Can you work these out from the model? Positions are in its coordinate system, mm. Face numbers are marked on the shaded views. Round coordinates to 2 decimals unless told otherwise and drop trailing zeros. Loops run counter-clockwise (first coordinate to the right, second up) from the corner with the lowest first, then second, coordinate; pieces in that order, holes last.
(1) I want a section at A-A on x = 152. Write out the boundary of the cut face in (y, z).
(2) If I drill on line 1 along Z through (x, y) = (158.5, 7.5); line 2 along X through (y, z) = (1.6, -30); line 3 along Z through (x, y) = (61, 8), over which ranges is the centre line in solid material (lowest first)?
(3) Thinking about a two-plate mould opening in X: for the marked faces 1, 2, 3 and 4, which applies, released by +X, released by -X, zero draft, split by the parting line, or undercut?
(4) I want a section at B-B on y = 9.5. Give the number of separate pieces and of enclosed holes in the cut face, plus the area to 3 significant figures.
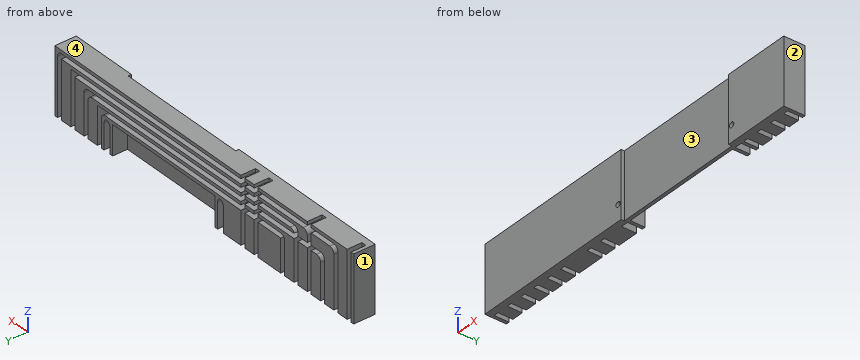
from build123d import *

# Parameters (mm, degrees)
PROFILESKETCH1_W              = 225
PROFILESKETCH1_H              = 40
PROFILEBOSS_EXTRUDE1_DEPTH    = 13
CABLE_GUIDESSKETCH2_W         = 27
CABLE_GUIDESSKETCH2_H         = 2
CABLE_GUIDESSKETCH2_W_2       = 7
CABLE_GUIDESSKETCH2_W_3       = 3
CABLE_GUIDESSKETCH2_H_2       = 40
CABLE_GUIDESSKETCH2_W_4       = 4.5
CABLE_GUIDESSKETCH2_H_3       = 18
CABLE_GUIDESSKETCH2_W_5       = 77
CABLEGUIDESCUT_EXTRUDE1_DEPTH = 9
FILLET3_R                     = 3
FILLET5_R                     = 3
FILLET6_R                     = 3
FILLET7_R                     = 3
BRIDGESKETCH2_W               = 81
BRIDGESKETCH2_H               = 2
BRIDGECUT_EXTRUDE3_DEPTH      = 229.897356909
MOUNTHOLESSKETCH4_R           = 1.592048555
MOUNTHOLESSKETCH4_R_2         = 1.651770992
MOUNTHOLESCUT_EXTRUDE4_DEPTH  = 229.705050228


with BuildPart() as part:
    # ProfileSketch1 → ProfileBoss-Extrude1 (new body)
    with BuildSketch(Plane(origin=(0, 0, 0), x_dir=(1, 0, 0), z_dir=(0, 1, 0))):
        with Locations((112.5, 20)):
            Rectangle(PROFILESKETCH1_W, PROFILESKETCH1_H)
    extrude(amount=PROFILEBOSS_EXTRUDE1_DEPTH)

    # Cable GuidesSketch2 → CableGuidesCut-Extrude1 (cut)
    # profile 1 of 5: a face of its own
    with BuildSketch(Plane(origin=(0, 13, 0), x_dir=(1, 0, 0), z_dir=(0, 1, 0))):
        Polygon((223, 2), (85, 2), (85, 0), (82, 0), (82, 2), (75, 2), (75, 0), (72, 0), (72, 2), (35, 2), (35, 0), (32, 0), (32, 2), (12, 2), (12, 40), (15, 40), (15, 5), (32, 5), (32, 12), (22, 12), (22, 40), (25, 40), (25, 15), (32, 15), (32, 40), (35, 40), (35, 15), (42, 15), (42, 40), (45, 40), (45, 15), (72, 15), (72, 17), (52, 17), (52, 40), (55, 40), (55, 20), (72, 20), (72, 40), (75, 40), (75, 20), (82, 20), (82, 40), (85, 40), (85, 20), (190, 20), (190, 40), (193, 40), (193, 17), (85, 17), (85, 15), (200, 15), (200, 40), (203, 40), (203, 12), (85, 12), (85, 10), (210, 10), (210, 40), (213, 40), (213, 7), (85, 7), (85, 5), (220, 5), (220, 40), (223, 40), align=None)
        Polygon((42, 7), (72, 7), (72, 5), (35, 5), (35, 12), (42, 12), align=None, mode=Mode.SUBTRACT)
        with Locations((58.5, 11)):
            Rectangle(CABLE_GUIDESSKETCH2_W, CABLE_GUIDESSKETCH2_H, mode=Mode.SUBTRACT)
        with Locations((78.5, 16)):
            Rectangle(CABLE_GUIDESSKETCH2_W_2, CABLE_GUIDESSKETCH2_H, mode=Mode.SUBTRACT)
        with Locations((78.5, 11)):
            Rectangle(CABLE_GUIDESSKETCH2_W_2, CABLE_GUIDESSKETCH2_H, mode=Mode.SUBTRACT)
        with Locations((78.5, 6)):
            Rectangle(CABLE_GUIDESSKETCH2_W_2, CABLE_GUIDESSKETCH2_H, mode=Mode.SUBTRACT)
    # profile 2 of 5: a face of its own
    with BuildSketch(Plane(origin=(0, 13, 0), x_dir=(1, 0, 0), z_dir=(0, 1, 0))):
        with Locations((3.5, 20)):
            Rectangle(CABLE_GUIDESSKETCH2_W_3, CABLE_GUIDESSKETCH2_H_2)
    # profile 3 of 5: a face of its own
    with BuildSketch(Plane(origin=(0, 13, 0), x_dir=(1, 0, 0), z_dir=(0, 1, 0))):
        with Locations((100.25, 31)):
            Rectangle(CABLE_GUIDESSKETCH2_W_4, CABLE_GUIDESSKETCH2_H_3)
    # profile 4 of 5: a face of its own
    with BuildSketch(Plane(origin=(0, 13, 0), x_dir=(1, 0, 0), z_dir=(0, 1, 0))):
        with Locations((185.75, 31)):
            Rectangle(CABLE_GUIDESSKETCH2_W_4, CABLE_GUIDESSKETCH2_H_3)
    # profile 5 of 5: a face of its own
    with BuildSketch(Plane(origin=(0, 13, 0), x_dir=(1, 0, 0), z_dir=(0, 1, 0))):
        with Locations((143, 31)):
            Rectangle(CABLE_GUIDESSKETCH2_W_5, CABLE_GUIDESSKETCH2_H_3)
    extrude(amount=-CABLEGUIDESCUT_EXTRUDE1_DEPTH, mode=Mode.SUBTRACT)

    # Fillet3
    fillet3_edges = [part.edges().sort_by_distance(p)[0] for p in [
        (183.5, 8.5, -22),
        (12, 8.5, -2),
        (22, 8.5, -12),
        (52, 8.5, -17),
        (42, 8.5, -7),
        (98, 8.5, -22),
    ]]
    fillet(fillet3_edges, radius=FILLET3_R)

    # Fillet5
    # the kernel refuses this fillet: 3 mm, written as the material it adds along each edge
    with BuildSketch(Plane(origin=(188, 13, -22), x_dir=(0, 0, -1), z_dir=(0, -1, 0)), Plane(origin=(102.5, 13, -22), x_dir=(0, 0, -1), z_dir=(0, -1, 0))) as fillet5_piece_1:
        with BuildLine():
            CenterArc((2.598076211, -3), FILLET5_R, 90, 60)
            Line((0, -1.5), (0, 0))
            Line((0, 0), (2.598076211, 0))
        make_face()
    extrude(amount=9)
    # the kernel refuses this fillet: 3 mm, written as the material it takes off along each edge
    with BuildSketch(Plane(origin=(200, 20.5, -15), x_dir=(0, 0, -1), z_dir=(0, -1, 0)), Plane(origin=(190, 20.5, -20), x_dir=(0, 0, -1), z_dir=(0, -1, 0))) as fillet5_2_piece_1:
        with BuildLine():
            CenterArc((FILLET5_R, -FILLET5_R), FILLET5_R, 90, 90)
            Line((0, -FILLET5_R), (0, 0))
            Line((0, 0), (FILLET5_R, 0))
        make_face()
    extrude(amount=16.5, mode=Mode.SUBTRACT)

    # Fillet6
    fillet6_edges = [part.edges().sort_by_distance(p)[0] for p in [
        (223, 8.5, -2),
        (203, 8.5, -12),
    ]]
    fillet(fillet6_edges, radius=FILLET6_R)

    # Fillet7
    # the kernel refuses this fillet: 3 mm, written as the material it takes off along each edge
    with BuildSketch(Plane(origin=(35, 20.5, -5), x_dir=(0, 0, -1), z_dir=(0, -1, 0)), Plane(origin=(15, 20.5, -5), x_dir=(0, 0, -1), z_dir=(0, -1, 0)), Plane(origin=(25, 20.5, -15), x_dir=(0, 0, -1), z_dir=(0, -1, 0))) as fillet7_piece_1:
        with BuildLine():
            CenterArc((FILLET7_R, FILLET7_R), FILLET7_R, 180, 90)
            Line((0, FILLET7_R), (-FILLET7_R * 0.02, FILLET7_R))
            Line((-FILLET7_R * 0.02, FILLET7_R), (-FILLET7_R * 0.02, -FILLET7_R * 0.02))
            Line((-FILLET7_R * 0.02, -FILLET7_R * 0.02), (FILLET7_R, -FILLET7_R * 0.02))
            Line((FILLET7_R, -FILLET7_R * 0.02), (FILLET7_R, 0))
        make_face()
    extrude(amount=16.5, mode=Mode.SUBTRACT)
    with BuildSketch(Plane(origin=(45, 20.071067812, -10), x_dir=(1, 0, 0), z_dir=(0, -1, 0))) as fillet7_piece_2:
        with BuildLine():
            CenterArc((2.828427125, -3), FILLET7_R, 90, 70.528779366)
            Line((0, -2), (-0.056568542, -1.98))
            ThreePointArc((-0.056568542, -1.98), (-0.06, -1), (-0.06, 0))
            Line((-0.06, 0), (0, 0.06))
            Line((0, 0.06), (2.828427125, 0.06))
            Line((2.828427125, 0.06), (2.828427125, 0))
        make_face()
    extrude(amount=16.071067812, mode=Mode.SUBTRACT)

    # BridgeSketch2 → BridgeCut-Extrude3 (cut, through all)
    with BuildSketch(Plane.XY):
        with Locations((143, 1)):
            Rectangle(BRIDGESKETCH2_W, BRIDGESKETCH2_H)
    extrude(amount=-BRIDGECUT_EXTRUDE3_DEPTH, mode=Mode.SUBTRACT)

    # MountHolesSketch4 → MountHolesCut-Extrude4 (cut, through all)
    with BuildSketch(Plane(origin=(0, 4, 0), x_dir=(1, 0, 0), z_dir=(0, 1, 0))):
        with Locations(Location((100.25, 30.227770246, 0), (0, 0, 270))):
            Circle(MOUNTHOLESSKETCH4_R)
        with Locations(Location((185.75, 30, 0), (0, 0, 270))):
            Circle(MOUNTHOLESSKETCH4_R_2)
    extrude(amount=-MOUNTHOLESCUT_EXTRUDE4_DEPTH, mode=Mode.SUBTRACT)


solid = part.part
Filled sheet:
1. outline: (2, -40) - (4, -40) - (4, -22) - (13, -22) - (13, -20) - (4, -20) - (4, -17) - (13, -17) - (13, -15) - (4, -15) - (4, -12) - (13, -12) - (13, -10) - (4, -10) - (4, -7) - (13, -7) - (13, -5) - (4, -5) - (4, -2) - (13, -2) - (13, 0) - (2, 0) - close
2. line 1: z = -22 to -20, -17 to -15, -12 to -10, -7 to -5, -2 to 0
2. line 2: x = 0 to 98.67, 101.83 to 102.5, 183.5 to 184.1, 187.4 to 225
2. line 3: z = -40 to -20, -17 to -15, -12 to -10, -7 to -5, -2 to 0
3. face 1: released by -X
3. face 2: released by +X
3. face 3: undercut
3. face 4: zero draft
4. separate pieces: 20
4. enclosed holes: 0
4. area: 4,310 mm2
